Could you check a few things on this model? Use its own coordinates, in mm. A direction names the side the tool comes from. Round coordinates to 2 decimals unless told otherwise and drop trailing zeros. Loops run counter-clockwise (first coordinate to the right, second up) from the corner with the lowest first, then second, coordinate; pieces in that order, holes last.
Autodesk Inventor part; units mm, degrees
ref_plane "YZ Plane" through (0, 0, 0) normal (1, 0, 0) x (0, 1, 0)
ref_plane "XZ Plane" through (0, 0, 0) normal (0, 1, 0) x (-1, 0, 0)
ref_plane "XY Plane" through (0, 0, 0) normal (0, 0, 1) x (1, 0, 0)
sketch "スケッチ3" plane through (0, 0, 0) normal (1, 0, 0) x (0, 1, 0)
  line L0 (0, 0) -> (0, -150)
  line L1 (0, 0) -> (0, -100)
  arc A0 (0, -150) -> (35.3553, -135.3553) centre (20.7107, -150) ccw
  line L2 (0, -150) -> (20.7107, -150) construction
  line L3 (35.3553, -135.3553) -> (20.7107, -150) construction
  line L4 (35.3553, -135.3553) -> (0, -100)
  line L5 (0, 0) -> (1, 0)
  arc A1 (1, -150) -> (34.6482, -136.0624) centre (20.7107, -150) ccw
  line L6 (34.6482, -136.0624) -> (1, -102.4142)
  line L7 (1, -150) -> (1, -102.4142)
  dimension "d13" = 150
  dimension "d14" = 100
  dimension "d16" = 135
  dimension "d17" = 1
extrude "押し出し3" add sketch "スケッチ3" along normal blind 15
sketch "スケッチ4" plane through (0, 0, 0) normal (-1, 0, 0) x (0, 0, 1)
  line L0 (-100, 0) -> (-150, 0)
  line L1 (-100, 0) -> (0, 0)
  line L2 (0, 0) -> (0, 1)
  line L3 (0, 1) -> (-101, 1)
  line L4 (-135.3553, 35.3553) -> (-100, 0)
  line L5 (-101, 1) -> (-100, 0)
  dimension "d20" = 1
extrude "押し出し4" add sketch "スケッチ4" against normal blind 15
sketch "スケッチ5" plane through (15, 0, 0) normal (1, 0, 0) x (0, 0, -1)
  line L0 (0, 0) -> (150, 0)
  line L1 (0, 0) -> (-10, 0)
  line L2 (-10, 0) -> (-10, 1)
  line L3 (-10, 1) -> (0, 1)
  line L4 (0, 1) -> (0, 0)
  dimension "d23" = 10
  dimension "d24" = 1
extrude "押し出し5" add sketch "スケッチ5" against normal blind 15
hole "穴1" at (7.5, 0, 3) direction (0, 1, 0) diameter 2.4 end through all
hole "穴2" at (7.5, 0, -13) direction (0, 1, 0) diameter 2.4 end through all
properties part number "スタビライザ" material "アルミニウム"
Item 1: If I drill on line 1 along X through (y, z) = (0.55, -13); line 2 along Y through (x, z) = (12.75, -80.5); line 3 along Z through (x, y) = (7.5, 11), over which ranges is the centre line in solid material (lowest first)?
Results list:
line 1: x = 0 to 6.3, 8.7 to 15
line 2: y = 0 to 1
line 3: z = -168.29 to -167.15, -112.41 to -111
Item 2: If we section it at C-C, the plane z = -48: Please give me the cut outline in (x, y), then the cut area to 3 significant figures.
Results list:
outline: (0, 0) - (15, 0) - (15, 1) - (0, 1) - close
area: 15.0 mm2
Item 3: For faces 4 (the flat face through (8, 0, -71)), 5 (the flat face through (8, 1, -45)), 6 (the flat face through (7, 1, -127)), which set-ups out of +Z, -Z, +X, -X, +Y, -Y let a thin tool reach every point of the face, with its end or its side?
Results list:
face 4: +Z, -Z, +X, -X, -Y
face 5: +Z, +X, -X, +Y
face 6: +X, -X
Item 4: If we section it at A-A, the plane x = 4.75: Please give me the cut outline in (y, z), then the cut area to 3 significant figures.
Results list:
outline: (0, -150) arc R20.71 ccw (long way) to (35.36, -135.36) - (1, -101) - (1, 10) - (0, 10) - close; hole (1, -150) arc R19.71 ccw (long way) to (34.65, -136.06) - (1, -102.41) - close
area: 287 mm2
Item 5: If we section it at B-B, the plane y = 16: Please give me the cut outline in (x, z).
Results list:
outline: (0, -170.17) - (15, -170.17) - (15, -169.14) - (0, -169.14) - close; (0, -117.41) - (15, -117.41) - (15, -116) - (0, -116) - close
Item 6: We'd pull the mould along Z, two halves only. Please class faces 1 (the cylindrical face through (7.395, 28.751, -167.996)), 2 (the flat face through (7, 18, -118)), 3 (the flat face through (0, 5.5, -106.7)): released by +Z, released by -Z, zero draft, split by the parting line, or undercut.
Results list:
face 1: undercut
face 2: released by +Z
face 3: zero draft
Item 7: Will these pins go through, and if not, where does the flat tip stop? pin 1 (23.5 mm diameter, centred on y = 20.71, z = -150, fed in from +X); pin 2 (1 mm diameter, centred on x = 2, y = 35.5, fed in from -Z); pin 3 (4.5 mm diameter, centred on x = 8.5, z = -138, fed in from +Y); pin 4 (1.5 mm diameter, centred on x = 8.5, y = 33, fed in from +Z).
Results list:
pin 1: passes through
pin 2: stops at z = -164.99
pin 3: stops at y = 38.98
pin 4: stops at z = -132.25
Item 8: If we section it at D-D, the plane y = 24.5: Please give me the cut outline in (x, z), then the cut area to 3 significant figures.
Results list:
outline: (0, -170.36) - (15, -170.36) - (15, -169.34) - (0, -169.34) - close; (0, -125.91) - (15, -125.91) - (15, -124.5) - (0, -124.5) - close
area: 36.5 mm2
